```python
from build123d import *

# Parameters (mm, degrees)
F1_DEPTH = 25.4
F3_DEPTH = 20.32
F5_D     = 5.9944
F5_DEPTH = 5.08
F5_TIP   = 1.8008994473


with BuildPart() as f1:
    # F0 (on Top) → F1 (new body)
    with BuildSketch(Plane.XY):
        Polygon((45.0902102752, -75.5565545624), (87.979000811, 1.2709902791), (42.8887905359, 76.8275448415), (-45.0902102752, 75.5565545624), (-87.979000811, -1.2709902791), (-42.8887905359, -76.8275448415), align=None)
    extrude(amount=F1_DEPTH)

    # F2 (on face) → F3 (cut)
    with BuildSketch(Plane.XY.offset(25.4)):
        Polygon((-25.7429317854, 25.4460219294), (-34.9083673088, 41.3210219294), (-53.2392383556, 41.3210219294), (-62.404673879, 25.4460219294), (-53.2392383556, 9.5710219294), (-34.9083673088, 9.5710219294), align=None)
        Polygon((-9.1654355234, 35.0170438588), (9.1654355234, 35.0170438588), (18.3308710468, 50.8920438588), (9.1654355234, 66.7670438588), (-9.1654355234, 66.7670438588), (-18.3308710468, 50.8920438588), align=None)
        Polygon((25.7429317854, -25.4460219294), (34.9083673088, -41.3210219294), (53.2392383556, -41.3210219294), (62.404673879, -25.4460219294), (53.2392383556, -9.5710219294), (34.9083673088, -9.5710219294), align=None)
        Polygon((34.9083673088, 9.5710219294), (53.2392383556, 9.5710219294), (62.404673879, 25.4460219294), (53.2392383556, 41.3210219294), (34.9083673088, 41.3210219294), (25.7429317854, 25.4460219294), align=None)
        Polygon((-9.1654355234, -35.0170438588), (-18.3308710468, -50.8920438588), (-9.1654355234, -66.7670438588), (9.1654355234, -66.7670438588), (18.3308710468, -50.8920438588), (9.1654355234, -35.0170438588), align=None)
        Polygon((-34.9083673088, -9.5710219294), (-53.2392383556, -9.5710219294), (-62.404673879, -25.4460219294), (-53.2392383556, -41.3210219294), (-34.9083673088, -41.3210219294), (-25.7429317854, -25.4460219294), align=None)
    extrude(amount=-F3_DEPTH, mode=Mode.SUBTRACT)

    # F5
    with Locations(Plane.XY.offset(25.4)):
        with Locations((-39.0446968377, 56.39789626), (43.9692549407, 56.39789626), (-39.0446968377, -56.39789626), (45.3762710094, -56.39789626)):
            Hole(F5_D / 2, depth=F5_DEPTH)
            with Locations((0, 0, -(F5_DEPTH + F5_TIP / 2))):  # 118° drill point
                Cone(0, F5_D / 2, F5_TIP, mode=Mode.SUBTRACT)


solid = f1.part
```
Work out the finished part from the listing and answer in its coordinate system (mm). Round coordinates to 2 decimals unless told otherwise and drop trailing zeros. Write each loop counter-clockwise with the first axis right and the second up, starting at its lowest first coordinate (ties: lowest second). Pieces come first, ordered by that corner, then holes.
1) A cutting plane is placed at D-D on y = 45. Determine the outline of the cut face in (x, z), and give its area (3 significant figures).
2) A cutting plane is placed at C-C on z = 10. Give the number of separate pieces and of enclosed holes in the cut face, and give its area (3 significant figures).
3) A cutting plane is placed at B-B on y = 29. Determine the outline of the cut face in (x, z).
4) Flat-ended cylindrical pins translate along their axes: P1, Ø5, axis at x = -10, z = 19.5, coming from the -Y side; P2, Ø14.5, axis at x = 44, z = 18, coming from the -Y side; P3, Ø1.5, axis at y = 35.5, z = 19.5, coming from the -X side. Find the tip coordinate at first contact, or state that the pin passes through.
5) Consider probe 1 along Y at (x, z) = (31.5, 6.25); probe 2 along X at (y, z) = (58.5, 20.25); probe 3 along Y at (x, z) = (17.5, 18.5). Determine where each line is inside the solid, lowest interval first.
6) A cutting plane is placed at A-A on x = 1.5. Determine the outline of the cut face in (y, z).
Entries:
1. outline: (-62.15, 0) - (61.88, 0) - (61.88, 25.4) - (14.93, 25.4) - (14.93, 5.08) - (-14.93, 5.08) - (-14.93, 25.4) - (-62.15, 25.4) - close
1. area: 2,540 mm2
2. separate pieces: 1
2. enclosed holes: 6
2. area: 14,900 mm2
3. outline: (-71.08, 0) - (71.43, 0) - (71.43, 25.4) - (60.35, 25.4) - (60.35, 5.08) - (27.79, 5.08) - (27.79, 25.4) - (-27.79, 25.4) - (-27.79, 5.08) - (-60.35, 5.08) - (-60.35, 25.4) - (-71.08, 25.4) - close
4. P1: stops at y = -76.39
4. P2: stops at y = -75.68
4. P3: stops at x = -67.87
5. probe 1: y = -75.75 to -35.42, -15.47 to 15.47, 35.42 to 76.66
5. probe 2: x = -54.61 to -41.01, -37.08 to -13.94, 13.94 to 42, 45.94 to 53.83
5. probe 3: y = -75.96 to -52.33, -49.45 to 49.45, 52.33 to 76.46
6. outline: (-76.19, 0) - (76.23, 0) - (76.23, 25.4) - (66.77, 25.4) - (66.77, 5.08) - (35.02, 5.08) - (35.02, 25.4) - (-35.02, 25.4) - (-35.02, 5.08) - (-66.77, 5.08) - (-66.77, 25.4) - (-76.19, 25.4) - close
